```python
from build123d import *

# Parameters (mm, degrees)
SKETCH2_W         = 4.2164
SKETCH2_H         = 22.352
CIRPATTERN1_COUNT = 20


with BuildPart() as part:
    # Sketch1 → Revolve1 (revolve)
    with BuildSketch(Plane.XY):
        Polygon((101.219, 11.176), (101.219, -11.176), (76.073, -11.176), (76.073, 10.852161676), (82.296, 10.852161676), (82.296, 10.541), (85.725, 9.292946067), (85.725, 11.176), align=None)
    revolve(axis=Axis((0, 42.36922773, 0), (0, -1, 0)))

    # Sketch2 → Cut-Revolve1 (revolve, cut)
    with BuildSketch(Plane.XY):
        with Locations((92.6338, 0)):
            Rectangle(SKETCH2_W, SKETCH2_H)
    cut_revolve1 = revolve(axis=Axis((90.5256, 40.326048615, 0), (0, -1, 0)), mode=Mode.SUBTRACT)

    # CirPattern1: Cut-Revolve1 ×20 about axis
    cirpattern1_axis = Axis((0, 0, 0), (0, 1, 0))
    for i in range(1, CIRPATTERN1_COUNT):
        add(cut_revolve1.rotate(cirpattern1_axis, i * 360 / CIRPATTERN1_COUNT), mode=Mode.SUBTRACT)


solid = part.part
```
For this review, take the finished solid that the model builds, in its own axes (mm). A direction names the side the tool comes from. Round coordinates to 2 decimals unless told otherwise and drop trailing zeros. Write each loop counter-clockwise with the first axis right and the second up, starting at its lowest first coordinate (ties: lowest second). Pieces come first, ordered by that corner, then holes. Notation, with made-up numbers: (77, 76.5) - (105, 76.5) arc R20 ccw to (105, 95.5) - close; hole circle Ø4 at (32.25, -9.75). An arc over 180 degrees is marked (long way). Use CSV: the item, a comma, the result in double quotes.
1) The part is to be moulded in two halves that separate along Z. For faces 3 (the flat face through (-73, 10.852, -24)), 4 (the flat face through (15, -11.176, 75)), say which applies: pulls with the +Z half, pulls with the -Z half, needs draft (parallel to the pull), parting line crosses it, or undercut.
Conclusion:
face 3,"undercut"
face 4,"needs draft"
2) For faces 1 (the cylindrical face through (-72.398, 0.156, 49.078)), 2 (the cylindrical face through (-10.713, 10.694, 81.596)), list the 3-axis set-ups (+Z, -Z, +X, -X, +Y, -Y) from which the entire face can be reached by the end or side of a thin tool; tool diameter is ignored.
Conclusion:
face 1,"+Y, -Y"
face 2,"+Y"
3) Add section A-A on z = 0. Write out the cut boundary in (x, y) (3 decimals), and give its area (3 significant figures).
Conclusion:
outline,"(-101.219, -11.176) - (-94.742, -11.176) - (-94.742, 11.176) - (-101.219, 11.176) - close; (-86.309, -11.176) - (-76.073, -11.176) - (-76.073, 10.852) - (-82.296, 10.852) - (-82.296, 10.541) - (-85.725, 9.293) - (-85.725, 11.176) - (-86.309, 11.176) - close; (76.073, -11.176) - (86.309, -11.176) - (86.309, 11.176) - (85.725, 11.176) - (85.725, 9.293) - (82.296, 10.541) - (82.296, 10.852) - (76.073, 10.852) - close; (94.742, -11.176) - (101.219, -11.176) - (101.219, 11.176) - (94.742, 11.176) - close"
area,"734 mm^2"
4) Add section B-B on x = 0. Write out the cut boundary in (y, z) (3 decimals), and give its area (3 significant figures).
Conclusion:
outline,"(-11.176, -101.219) - (11.176, -101.219) - (11.176, -94.742) - (-11.176, -94.742) - close; (-11.176, -86.309) - (11.176, -86.309) - (11.176, -85.725) - (9.293, -85.725) - (10.541, -82.296) - (10.852, -82.296) - (10.852, -76.073) - (-11.176, -76.073) - close; (-11.176, 76.073) - (10.852, 76.073) - (10.852, 82.296) - (10.541, 82.296) - (9.293, 85.725) - (11.176, 85.725) - (11.176, 86.309) - (-11.176, 86.309) - close; (-11.176, 94.742) - (11.176, 94.742) - (11.176, 101.219) - (-11.176, 101.219) - close"
area,"734 mm^2"
5) Clearance check with flat-ended pins moving along their axes: pin 1 Ø4 at (x, y) = (46, 4) entering from -Z; pin 2 Ø6 at (y, z) = (2.5, -10.5) entering from +X; pin 3 Ø1.5 at (y, z) = (8, -63) entering from -X. State where each tip first meets the part, or that it passes through.
Conclusion:
pin 1,"stops at z = -91.16"
pin 2,"stops at x = 100.94"
pin 3,"stops at x = -79.81"
6) Add section C-C on y = 1. Count the separate pieces of the cut face and the enclosed holes in it, and give its area (3 significant figures).
Conclusion:
separate pieces,"1"
enclosed holes,"21"
area,"12,900 mm^2"
7) Wall thickness on line 1 along Z through (x, y) = (-1.5, -4.25); line 2 along X through (y, z) = (3.25, -86); line 3 along Z through (x, y) = (-76.5, -3.25): over which ranges is each line inside the solid? List them lowest first. Write a range as from..to.
Conclusion:
line 1,"z = -101.21..-94.47, -86.59..-76.06, 76.06..86.59, 94.47..101.21"
line 2,"x = -53.38..-32.19, -23.76..23.76, 32.19..53.38"
line 3,"z = -66.28..-55.88, -50.54..50.54, 55.88..66.28"
